from build123d import *

# Parameters (mm, degrees)
SKETCH1_R      = 1.5
EXTRUDE1_DEPTH = 2
FILLET1_R      = 3
FILLET2_R      = 3.5
EXTRUDE2_DEPTH = 2
EXTRUDE3_DEPTH = 2
FILLET3_R      = 3
FILLET5_R      = 7


with BuildPart() as part:
    # Sketch1 → Extrude1 (new body)
    # profile 1 of 2: a face of its own
    with BuildSketch(Plane(origin=(0, 0, 0), x_dir=(1, 0, 0), z_dir=(0, 1, 0))):
        Polygon((-22, 0), (0, 0), (0, 7), (-29, 7), (-29, -18), (-22, -18), align=None)
        with Locations(Location((-25.5, -14.5, 0), (0, 0, 270))):
            Circle(SKETCH1_R, mode=Mode.SUBTRACT)
        with Locations(Location((-11, 3.5, 0), (0, 0, 270))):
            Circle(SKETCH1_R, mode=Mode.SUBTRACT)
    # profile 2 of 2: a face of its own
    with BuildSketch(Plane(origin=(0, 0, 0), x_dir=(1, 0, 0), z_dir=(0, 1, 0))):
        Polygon((0, 0), (22, 0), (22, -18), (29, -18), (29, 7), (0, 7), align=None)
        with Locations(Location((25.5, -14.5, 0), (0, 0, 270))):
            Circle(SKETCH1_R, mode=Mode.SUBTRACT)
        with Locations(Location((11, 3.5, 0), (0, 0, 270))):
            Circle(SKETCH1_R, mode=Mode.SUBTRACT)
    extrude(amount=EXTRUDE1_DEPTH)

    # Fillet1
    fillet1_edges = [part.edges().sort_by_distance(p)[0] for p in [
        (-22, 1, 0),
        (22, 1, 0),
    ]]
    fillet(fillet1_edges, radius=FILLET1_R)

    # Fillet2
    fillet2_edges = [part.edges().sort_by_distance(p)[0] for p in [
        (29, 1, 18),
        (22, 1, 18),
        (-22, 1, 18),
        (-29, 1, 18),
    ]]
    fillet(fillet2_edges, radius=FILLET2_R - 0.0001)  # a hair under: the kernel refuses the full size

    # Sketch2 → Extrude2 (cut)
    with BuildSketch(Plane(origin=(0, 2, 0), x_dir=(1, 0, 0), z_dir=(0, 1, 0))):
        with BuildLine():
            Line((-9.5, 7), (9.5, 7))
            add(Edge.make_bspline(
                [(-9.5, 7), (-9.5, 5.5), (0, 5.5), (9.5, 5.5), (9.5, 7)],
                knots=[0, 0, 0, 1.570796327, 1.570796327, 3.141592654, 3.141592654, 3.141592654], degree=2, weights=[1, 0.707106781, 1, 0.707106781, 1]))
        make_face()
    extrude2 = extrude(amount=-EXTRUDE2_DEPTH, mode=Mode.SUBTRACT)

    # Mirror1: Extrude2 across plane
    add(extrude2.mirror(Plane(origin=(0, 0, -3.5), x_dir=(1, 0, 0), z_dir=(0, 0, -1))), mode=Mode.SUBTRACT)

    # Sketch3 → Extrude3 (cut)
    with BuildSketch(Plane(origin=(0, 2, 0), x_dir=(-1, 0, 0), z_dir=(0, 1, 0))):
        with BuildLine():
            Line((-13, 0), (-19, 0))
            ThreePointArc((-19, 0), (-21.121320344, 0.878679656), (-22, 3))
            Line((-22, 3), (-22, 9))
            ThreePointArc((-22, 9), (-23.031608424, -1.031608424), (-13, 0))
        make_face()
    extrude3 = extrude(amount=-EXTRUDE3_DEPTH, mode=Mode.SUBTRACT)

    # Mirror4: Extrude3 across plane
    add(extrude3.mirror(Plane(origin=(0, 0, 0), x_dir=(0, 0, 1), z_dir=(1, 0, 0))), mode=Mode.SUBTRACT)

    # Fillet3
    fillet3_edges = [part.edges().sort_by_distance(p)[0] for p in [
        (9.5, 1, 0),
        (-9.5, 1, 0),
        (22, 1, 9),
        (13, 1, 0),
        (-9.5, 1, -7),
        (9.5, 1, -7),
        (-22, 1, 9),
        (-13, 1, 0),
    ]]
    fillet(fillet3_edges, radius=FILLET3_R)

    # Fillet5
    fillet5_edges = [part.edges().sort_by_distance(p)[0] for p in [
        (-29, 1, -7),
        (29, 1, -7),
    ]]
    fillet(fillet5_edges, radius=FILLET5_R)


solid = part.part
Input: part model. Units: mm. Frame: model coordinates. A direction names the side the tool comes from. Round coordinates to 2 decimals unless told otherwise and drop trailing zeros. Loops run counter-clockwise (first coordinate to the right, second up) from the corner with the lowest first, then second, coordinate; pieces in that order, holes last. Notation, with made-up numbers: (-8.75, -25.75) -> (20.25, -25.75) arc R35 ccw to (20.25, 12.25) -> close; hole circle Ø3 at (-11, 53.25). An arc over 180 degrees is marked (long way). Answer as a JSON object with one key per item and string values. Group by question number.
1) Section query B-B on y = 1.6. State how many separate pieces and enclosed holes the cut face has, plus the area to 3 significant figures.
2) Section query A-A on z = 11.5. Output: boundary loops of the cut face in (x, y).
3) Pin query (flat end, axial travel): pin 1 (0.5 mm diameter, centred on x = 11, y = 1, fed in from +Z). Return the tip coordinate at first contact, or that it passes through.
4) Ray query, L1, parallel to X at y = 1.5, z = 14.5; L2, parallel to X at y = 1.15, z = -3.5; L3, parallel to X at y = 0.2, z = 15. Return the intervals inside material, ascending.
5) Draft query along Z for faces 1 (the cylindrical face through (27, 1, -4.9)), 2 (the cylindrical face through (-22.248, 0.986, 9.237)), 3 (the cylindrical face through (27.95, 1.01, 17)). Return one class per face: +Z half, -Z half, draft (parallel to the pull), parting line (faces both ways), or undercut.
6) Reachability of faces 4 (the cylindrical face through (-28, 1.01, 16.95)), 5 (the cylindrical face through (23, 1.01, 16.95)), 6 (the cylindrical face through (22.248, 0.986, 9.237)) from +Z, -Z, +X, -X, +Y, -Y: full face, straight path, thin tool, end or side. Return the list, or none.
7) Section query C-C on x = 20. Output: boundary loops of the cut face in (y, z), plus the area to 3 significant figures.
Reply:
{
 "1": {"separate pieces": "1", "enclosed holes": "4", "area": "466 mm2"},
 "2": {"outline": "(-29, 0) -> (-22, 0) -> (-22, 2) -> (-29, 2) -> close; (22, 0) -> (29, 0) -> (29, 2) -> (22, 2) -> close"},
 "3": {"pin 1": "stops at z = 0"},
 "4": {"L1": "x = -29 to -27, -24 to -22, 22 to 24, 27 to 29", "L2": "x = -28.06 to -12.5, -9.5 to 9.5, 12.5 to 28.06", "L3": "x = -28.96 to -26.91, -24.09 to -22.04, 22.04 to 24.09, 26.91 to 28.96"},
 "5": {"face 1": "-Z half", "face 2": "undercut", "face 3": "+Z half"},
 "6": {"face 4": "+Z, -X, +Y, -Y", "face 5": "+Z, +Y, -Y", "face 6": "+Y, -Y"},
 "7": {"outline": "(0, -7) -> (2, -7) -> (2, -2.74) -> (0, -2.74) -> close", "area": "8.51 mm2"}
}
